Here's how the part is built. I have some questions about the finished solid (model axes, mm). A direction names the side the tool comes from. Round coordinates to 2 decimals unless told otherwise and drop trailing zeros. Order: outer loops, then holes, each group sorted by start corner. A loop starts at its lowest first (then second) coordinate and runs counter-clockwise, first axis right, second up. Notation, with made-up numbers: (78.5, -31.5) -> (130.5, -31.5) arc R14 ccw to (130.5, -25.5) -> close; hole circle Ø3 at (46, 52). An arc over 180 degrees is marked (long way). Use a Markdown table: item, result. Add a question column.
from build123d import *

# Parameters (mm, degrees)
F0_W      = 177.8
F0_H      = 50.8
F1_DEPTH  = 69.85
F3_DEPTH  = 50.8
F2_R      = 22.225
F4_DEPTH  = 50.8
F5_DEPTH  = 50.8
F7_DEPTH  = 50.8
F6_R      = 12.7
F8_DEPTH  = 50.8
F10_DEPTH = 50.8
F12_DEPTH = 28.575
F13_R     = 22.225
F14_DEPTH = 12.7


# Not quite as in the source:
# - ends of sketch curves that miss each other by under 0.0002 mm in the source are joined


with BuildPart() as f1:
    # F0 (on Front) → F1 (new body)
    with BuildSketch(Plane.XZ):
        with Locations((88.9, 25.4)):
            Rectangle(F0_W, F0_H)
    extrude(amount=F1_DEPTH)

    # F2 (on face) → F3 (cut, through all)
    with BuildSketch(Plane.XY.offset(50.8)):
        with BuildLine():
            Line((0, -69.85), (34.925, -69.85))
            ThreePointArc((34.925, -69.85), (10.2292956671, -59.6207043329), (0, -34.925))
            Line((0, -34.925), (0, -69.85))
        make_face()
        with BuildLine():
            ThreePointArc((0, -34.925), (10.2292957417, -10.2292955924), (34.9250002112, 0))
            Line((34.9250002112, 0), (0, 0))
            Line((0, 0), (0, -34.925))
        make_face()
    extrude(amount=-F3_DEPTH, mode=Mode.SUBTRACT)

    # F2 (on face) → F4 (cut, through all)
    with BuildSketch(Plane.XY.offset(50.8)):
        with Locations((34.925, -34.925)):
            Circle(F2_R)
    extrude(amount=-F4_DEPTH, mode=Mode.SUBTRACT)

    # F5 (add): a face of the model
    f5_faces = [f1.faces().sort_by_distance(p)[0] for p in [
        (177.8, -34.925, 25.4),
    ]]
    extrude(f5_faces, amount=F5_DEPTH)

    # F6 (on face) → F7 (cut, through all)
    with BuildSketch(Plane.XY.offset(50.8)):
        with BuildLine():
            Line((228.6, 0), (34.9250002112, 0))
            Line((34.9250002112, 0), (180.975, -10.3535739202))
            ThreePointArc((180.975, -10.3535739202), (203.8662068568, -34.925), (180.975, -59.4964260798))
            Line((180.975, -59.4964260798), (34.925, -69.85))
            Line((34.925, -69.85), (228.6, -69.85))
            Line((228.6, -69.85), (228.6, 0))
        make_face()
    extrude(amount=-F7_DEPTH, mode=Mode.SUBTRACT)

    # F6 (on face) → F8 (cut, through all)
    with BuildSketch(Plane.XY.offset(50.8)):
        with Locations((179.2331165612, -34.925)):
            Circle(F6_R)
    extrude(amount=-F8_DEPTH, mode=Mode.SUBTRACT)

    # F9 (on face) → F10 (cut, through all)
    with BuildSketch(Plane.XY.offset(50.8)):
        with BuildLine():
            ThreePointArc((179.2331165612, -12.7), (194.948564773, -19.2095517881), (201.4581165612, -34.925))
            ThreePointArc((201.4581165612, -34.925), (194.948564773, -50.6404482119), (179.2331165612, -57.15))
            Line((179.2331165612, -57.15), (34.925, -69.85))
            Line((34.925, -69.85), (180.975, -59.4964260798))
            ThreePointArc((180.975, -59.4964260798), (203.8662068568, -34.925), (180.975, -10.3535739202))
            Line((180.975, -10.3535739202), (34.9250002112, 0))
            Line((34.9250002112, 0), (179.2331165612, -12.7))
        make_face()
    extrude(amount=-F10_DEPTH, mode=Mode.SUBTRACT)

    # F11 (on face) → F12 (cut)
    with BuildSketch(Plane.XY.offset(50.8)):
        with BuildLine():
            ThreePointArc((40.4881105931, -0.4895878599), (69.5805320507, -34.9249998886), (40.4881108127, -69.3604121029))
            Line((40.4881108127, -69.3604121029), (179.2331165612, -57.15))
            ThreePointArc((179.2331165612, -57.15), (157.0081165612, -34.925), (179.2331165612, -12.7))
            Line((179.2331165612, -12.7), (40.4881105931, -0.4895878599))
        make_face()
    extrude(amount=-F12_DEPTH, mode=Mode.SUBTRACT)

    # F13 (on face) → F14 (cut)
    with BuildSketch(Plane.XY.offset(50.8)):
        with Locations((179.2331165612, -34.925)):
            Circle(F13_R)
    extrude(amount=-F14_DEPTH, mode=Mode.SUBTRACT)


solid = f1.part
(1) I want a section at D-D on x = 54. List the corners of the cut face in (y, z) for me (3 decimals).
(2) Please list where these lines run through material, in increasing order: probe 1 along X at (y, z) = (-19.5, 26); probe 2 along X at (y, z) = (-27.5, 35); probe 3 along X at (y, z) = (-54.5, 25). Write a range as from..to.
(3) On a 3-axis mill with a long thin cutter (end or side, diameter ignored), from which of +Z, -Z, +X, -X, +Y, -Y can I reach the whole of each face in a straight line? I mean faces 4 (the cylindrical face through (166.545, -34.367, 19.317)), 5 (the cylindrical face through (69.574, -34.239, 36.713)), 6 (the flat face through (189, -44, 38.1)). Say none if no direction works.
(4) I'm going to push flat-ended pins straight in: P1, Ø12, axis at x = 89, z = 6, coming from the -Y side; P2, Ø8, axis at y = -39.5, z = 30.5, coming from the -X side; P3, Ø1, axis at y = -52, z = 23, coming from the +X side; P4, Ø20.5, axis at x = 179.23, y = -34.92, coming from the -Z side. Where does each tip first touch, or does it pass through?
(5) I want a section at B-B on z = 10.5. List the corners of the cut face in (x, y) for me (3 decimals), and give its area (3 significant figures).
(6) If we mould it in two halves opening along X, with no side actions, what happens to faces 1 (the flat face through (57.5, -34.4, 50.8)), 2 (the flat face through (106.07, -6.26, 14.47)), 3 (the cylindrical face through (12.72, -33.95, 25.76))? For each: pulls with the +X half, pulls with the -X half, needs draft (parallel to the pull), parting line crosses it, or undercut.
(7) I want a section at A-A on z = 25. List the corners of the cut face in (x, y) for me (3 decimals).
(8) I want a section at C-C on y = -27.5. List the corners of the cut face in (x, z) for me (3 decimals).
Output:
| question | item | result |
|---|---|---|
| 1 | outline | (-68.171, 0) -> (-46.331, 0) -> (-46.331, 50.8) -> (-64.004, 50.8) -> (-64.004, 22.225) -> (-68.171, 22.225) -> close; (-23.519, 0) -> (-1.679, 0) -> (-1.679, 22.225) -> (-5.846, 22.225) -> (-5.846, 50.8) -> (-23.519, 50.8) -> close |
| 2 | probe 1 | 3.59..18.92, 50.93..65.99, 163.23..195.23 |
| 2 | probe 2 | 0.8..13.98, 55.87..68.78, 158.29..168.93, 189.54..200.18 |
| 2 | probe 3 | 6..24.4, 45.45..63.58, 168.71..189.76 |
| 3 | face 4 | +Z, -Z |
| 3 | face 5 | +Z |
| 3 | face 6 | +Z, +X, +Y, -Y |
| 4 | P1 | y = -65.62 |
| 4 | P2 | x = 0 |
| 4 | P3 | x = 194.04 |
| 4 | P4 | through |
| 5 | outline | (34.925, -69.85) -> (179.233, -57.15) arc R22.225 ccw to (179.233, -12.7) -> (34.925, 0) arc R34.925 ccw to start; hole circle Ø44.45 at (34.925, -34.925); hole circle Ø25.4 at (179.233, -34.925) |
| 5 | area | 8,880 mm² |
| 6 | face 1 | needs draft |
| 6 | face 2 | pulls with the +X half |
| 6 | face 3 | undercut |
| 7 | outline | (34.925, -69.85) -> (40.488, -69.36) arc R34.926 ccw to (40.488, -0.49) -> (34.925, 0) arc R34.925 ccw to start; circle Ø44.45 at (179.233, -34.925); hole circle Ø44.45 at (34.925, -34.925); hole circle Ø25.4 at (179.233, -34.925) |
| 8 | outline | (0.798, 0) -> (13.977, 0) -> (13.977, 50.8) -> (0.798, 50.8) -> close; (55.873, 0) -> (168.93, 0) -> (168.93, 38.1) -> (158.285, 38.1) -> (158.285, 22.225) -> (68.782, 22.225) -> (68.782, 50.8) -> (55.873, 50.8) -> close; (189.536, 0) -> (200.181, 0) -> (200.181, 38.1) -> (189.536, 38.1) -> close |
